Here's how the part is built. I have some questions about the finished solid (model axes, mm). Face numbers are marked on the shaded views. A direction names the side the tool comes from. Give positions to 0.01 mm unless a question says otherwise; leave off trailing zeros. Loops run counter-clockwise (first coordinate to the right, second up) from the corner with the lowest first, then second, coordinate; pieces in that order, holes last. Notation, with made-up numbers: M 15,52 L 56,52 A19 ccw 56,73 Z; hole C 74.5,-31 d4. An arc over 180 degrees is marked long. Write item = value, one per line. Start each with the question number.
```python
from build123d import *

# Parameters (mm, degrees)
F0_R     = 20
F0_R_2   = 2.5
F0_R_3   = 7.5
F0_R_4   = 2.55
F1_DEPTH = 10
F2_DEPTH = 3
F3_R     = 0.5


with BuildPart() as f1:
    # F0 (on Top) → F1 (new body)
    with BuildSketch(Plane.XY):
        Circle(F0_R)
        with Locations((0, -15)):
            Circle(F0_R_2, mode=Mode.SUBTRACT)
        with Locations((-15, 0)):
            Circle(F0_R_2, mode=Mode.SUBTRACT)
        Circle(F0_R_3, mode=Mode.SUBTRACT)
        with Locations((15, 0)):
            Circle(F0_R_2, mode=Mode.SUBTRACT)
        with Locations((0, 15)):
            Circle(F0_R_2, mode=Mode.SUBTRACT)
        with Locations((-15, 0)):
            Circle(F0_R_2)
        Circle(F0_R_3)
        Circle(F0_R_4, mode=Mode.SUBTRACT)
        with Locations((15, 0)):
            Circle(F0_R_2)
        with Locations((0, -15)):
            Circle(F0_R_2)
        with Locations((0, 15)):
            Circle(F0_R_2)
    extrude(amount=F1_DEPTH)

    # F0 (on Top) → F2 (cut)
    with BuildSketch(Plane.XY):
        with Locations((0, 15)):
            Circle(F0_R_2)
        with Locations((-15, 0)):
            Circle(F0_R_2)
        with Locations((0, -15)):
            Circle(F0_R_2)
        with Locations((15, 0)):
            Circle(F0_R_2)
        Circle(F0_R_3)
        Circle(F0_R_4, mode=Mode.SUBTRACT)
    extrude(amount=F2_DEPTH, mode=Mode.SUBTRACT)

    # F3
    f3_edges = [f1.edges().sort_by_distance(p)[0] for p in [
        (-2.55, 0, 3),
        (-20, 0, 0),
        (-20, 0, 10),
    ]]
    fillet(f3_edges, radius=F3_R)


solid = f1.part
```
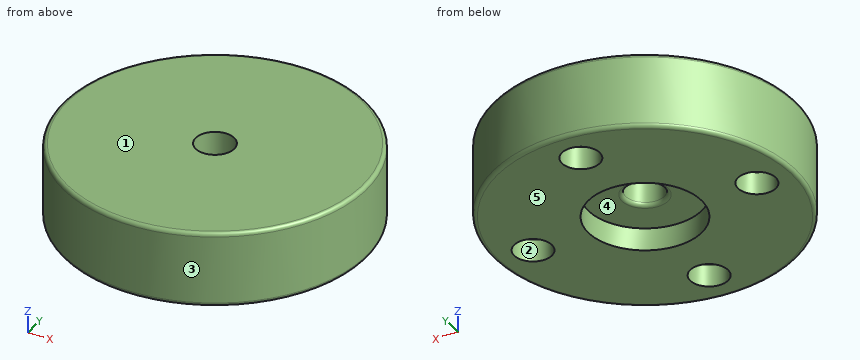
Q1. We'd pull the mould along Y, two halves only. Please class the marked faces 3, 4 and 5: pulls with the +Y half, pulls with the -Y half, needs draft (parallel to the pull), parting line crosses it, or undercut.
Q2. If we section it at B-B, the plane z = 1.5: List the corners of the cut face in (x, y) for me.
Q3. Will these pins go through, and if not, where does the flat tip stop? pin 1 (3 mm diameter, centred on x = 0.5, y = 3, fed in from -Z); pin 2 (6 mm diameter, centred on x = -4, z = 2, fed in from -Y) (3 decimals); pin 3 (1.5 mm diameter, centred on x = -12, z = 3, fed in from -Y).
Q4. If we section it at A-A, the plane y = 0: List the corners of the cut face in (x, z) for me, then the cut area to 3 significant figures.
Q5. If I drill on line 1 along Y through (x, z) = (0, 2.15); line 2 along Y through (x, z) = (-0.5, 4); line 3 along Z through (x, y) = (-2.5, -4.5), over which ranges is the centre line in solid material (lowest first)?
Q6. If we section it at D-D, the plane z = 8: List the corners of the cut face in (x, y) for me, then the cut area to 3 significant figures.
Q7. On a 3-axis mill with a long thin cutter (end or side, diameter ignored), from which of +Z, -Z, +X, -X, +Y, -Y can I reach the whole of each face in a straight line? I mean the marked faces 1 and 2. Say none if no direction works.
Resolved:
q1.face_3 = parting line crosses it
q1.face_4 = undercut
q1.face_5 = needs draft
q2.outline = C 0,0 d40; hole C -15,0 d5; hole C 0,0 d15; hole C 0,-15 d5; hole C 0,15 d5; hole C 15,0 d5
q3.pin_1 = 3
q3.pin_2 = -19.975
q3.pin_3 = -16.54
q4.outline = M -20,0.5 A0.5 ccw -19.5,0 L -17.5,0 L -17.5,3 L -12.5,3 L -12.5,0 L -7.5,0 L -7.5,3 L -3.05,3 A0.5 ccw -2.55,3.5 L -2.55,10 L -19.5,10 A0.5 ccw -20,9.5 Z; M 2.55,3.5 A0.5 ccw 3.05,3 L 7.5,3 L 7.5,0 L 12.5,0 L 12.5,3 L 17.5,3 L 17.5,0 L 19.5,0 A0.5 ccw 20,0.5 L 20,9.5 A0.5 ccw 19.5,10 L 2.55,10 Z
q4.area = 289 mm²
q5.line_1 = -20 to -17.5, -12.5 to -7.5, 7.5 to 12.5, 17.5 to 20
q5.line_2 = -19.99 to -2.5, 2.5 to 19.99
q5.line_3 = 3 to 10
q6.outline = C 0,0 d40; hole C 0,0 d5.1
q6.area = 1,240 mm²
q7.face_1 = +Z, +X, -X, +Y, -Y
q7.face_2 = -Z
